```python
from build123d import *

# Parameters (mm, degrees)
CYLINDER_R     = 1.5
CYLINDER_DEPTH = 10
BOX002_W       = 103
BOX002_H       = 1
BOX002_DEPTH   = 10
BOX003_W       = 103
BOX003_H       = 1
BOX003_DEPTH   = 20
BOX001_W       = 103
BOX001_H       = 49
BOX001_DEPTH   = 34
BOX_W          = 105
BOX_H          = 50
BOX_DEPTH      = 35


with BuildPart() as pump_hole:
    # Cylinder → Cylinder (new body)
    with BuildSketch(Plane(origin=(100, 33, 5), x_dir=(0, 0, -1), z_dir=(1, 0, 0))):
        Circle(CYLINDER_R)
    extrude(amount=CYLINDER_DEPTH)


with BuildPart() as front_piece:
    # Box002 → Box002 (new body)
    with BuildSketch(Plane(origin=(1, 0, 1), x_dir=(1, 0, 0), z_dir=(0, 0, 1))):
        with Locations((51.5, 0.5)):
            Rectangle(BOX002_W, BOX002_H)
    extrude(amount=BOX002_DEPTH)


with BuildPart() as mid_piece:
    # Box003 → Box003 (new body)
    with BuildSketch(Plane(origin=(1, 16, 1), x_dir=(1, 0, 0), z_dir=(0, 0, 1))):
        with Locations((51.5, 0.5)):
            Rectangle(BOX003_W, BOX003_H)
    extrude(amount=BOX003_DEPTH)


with BuildPart() as primary_cut_out:
    # Box001 → Box001 (new body)
    with BuildSketch(Plane(origin=(1, 0, 1), x_dir=(1, 0, 0), z_dir=(0, 0, 1))):
        with Locations((51.5, 24.5)):
            Rectangle(BOX001_W, BOX001_H)
    extrude(amount=BOX001_DEPTH)


with BuildPart() as pool:
    # Box → Box (new body)
    with BuildSketch(Plane.XY):
        with Locations((52.5, 25)):
            Rectangle(BOX_W, BOX_H)
    extrude(amount=BOX_DEPTH)

    # Cut: cut Primary Cut Out
    add(primary_cut_out.part, mode=Mode.SUBTRACT)

    # Fusion: union Front Piece, Mid Piece
    add(front_piece.part)
    add(mid_piece.part)

    # Cut001: cut Pump Hole
    add(pump_hole.part, mode=Mode.SUBTRACT)


with BuildPart() as pool_1:
    # Cut001 placement: moved
    add(pool.part.moved(Location((2, 0, 0))))


solid = pool_1.part
```
Geometry: final body of the model. Coordinates: model frame, mm. A direction names the side the tool comes from. Round coordinates to 2 decimals unless told otherwise and drop trailing zeros. Order: outer loops, then holes, each group sorted by start corner. A loop starts at its lowest first (then second) coordinate and runs counter-clockwise, first axis right, second up. Notation, with made-up numbers: M -2,14.5 L 22,14.5 A20 ccw 22,38.5 Z; hole C 44,79 d7. An arc over 180 degrees is marked long. Use one line per item in the form item = value. Start each with the question number.
Q1. Cut plane B-B (z = 13.5). Return loops of the section in (x, y).
Q2. Cut plane D-D (x = 79.5). Return loops of the section in (y, z).
Q3. Pin query (flat end, axial travel): pin 1 Ø12 at (x, y) = (77, 12) entering from +Z; pin 2 Ø2 at (x, y) = (36.5, 44) entering from -Z; pin 3 Ø2.5 at (y, z) = (33, 5) entering from +X; pin 4 Ø0.8 at (x, y) = (39.5, 0.5) entering from +Z. Return the tip coordinate at first contact, or that it passes through.
Q4. Cut plane C-C (z = 2). Return loops of the section in (x, y).
Q5. Material intervals for line 1 (Y direction, x = 93.5, z = 7); line 2 (X direction, y = 30, z = 15); line 3 (Y direction, x = 106.85, z = 5), sorted ascending. Write a range as [from, to].
Q6. Cut plane A-A (y = 33). Return loops of the section in (x, z), and give its area (3 significant figures).
Q7. Mould query, pull axis X, two halves, no side actions, for faces 4 (the face through (54, 17, 11)), 5 (the face through (107, 25, 17)), 6 (the face through (2, 25, 17)), 7 (the face through (54.3, 49.2, 35)). Classes: +X half, -X half, draft (parallel to the pull), parting line (faces both ways), or undercut.
Q8. Access query for faces 1 (the face through (106.493, 31.536, 5.325)), 2 (the face through (54, 49, 18)), 3 (the face through (54, 0, 4)). Directions: +Z, -Z, +X, -X, +Y, -Y. A direction counts if a zero-diameter tool reaches every point of the face in a straight line with its end or side. Return the directions, or none.
Geometry results:
q1.outline = M 2,0 L 3,0 L 3,16 L 106,16 L 106,0 L 107,0 L 107,50 L 2,50 Z; hole M 3,17 L 106,17 L 106,49 L 3,49 Z
q2.outline = M 0,0 L 50,0 L 50,35 L 49,35 L 49,1 L 17,1 L 17,21 L 16,21 L 16,1 L 1,1 L 1,11 L 0,11 Z
q3.pin_1 = 21
q3.pin_2 = 0
q3.pin_3 = 3
q3.pin_4 = 11
q4.outline = M 2,0 L 107,0 L 107,50 L 2,50 Z; hole M 3,1 L 106,1 L 106,16 L 3,16 Z; hole M 3,17 L 106,17 L 106,49 L 3,49 Z
q5.line_1 = [0, 1], [16, 17], [49, 50]
q5.line_2 = [2, 3], [106, 107]
q5.line_3 = [0, 31.5], [34.5, 50]
q6.outline = M 2,0 L 107,0 L 107,3.5 L 106,3.5 L 106,1 L 3,1 L 3,35 L 2,35 Z; M 106,6.5 L 107,6.5 L 107,35 L 106,35 Z
q6.area = 170 mm^2
q7.face_4 = undercut
q7.face_5 = +X half
q7.face_6 = -X half
q7.face_7 = draft
q8.face_1 = +X
q8.face_2 = +Z
q8.face_3 = +Z, -Z, +X, -X, -Y
